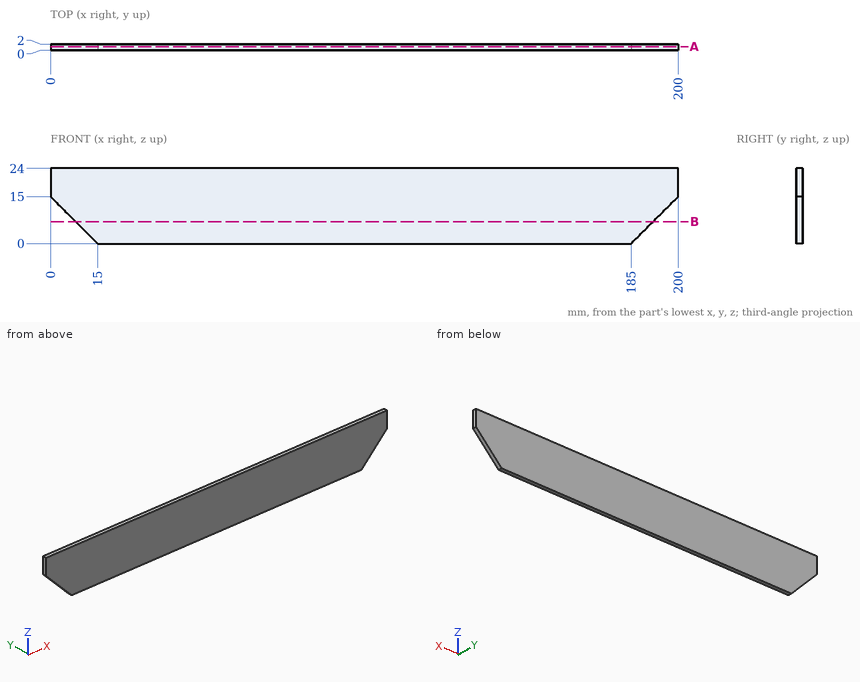
Print and shaded views of the part. All mm, measured from the part's lowest x, y and z. Give positions to 0.01 mm unless a question says otherwise; leave off trailing zeros. Loops run counter-clockwise (first coordinate to the right, second up) from the corner with the lowest first, then second, coordinate; pieces in that order, holes last.
1) Saw through at A-A (y = 1.15). Write the cut outline in (x, z), plus the area to 4 significant figures.
2) Saw through at B-B (z = 7). Write the cut outline in (x, y).
3) Wall check: line 1 (X direction, y = 1.2, z = 14); line 2 (Z direction, x = 14.5, y = 1.1); line 3 (X direction, y = 1.35, z = 10.5). Give the ranges that are in metal, low to high.
Answer block:
1. outline: (0, 15) - (15, 0) - (185, 0) - (200, 15) - (200, 24) - (0, 24) - close
1. area: 4,575 mm2
2. outline: (8, 0) - (192, 0) - (192, 2) - (8, 2) - close
3. line 1: x = 1 to 199
3. line 2: z = 0.5 to 24
3. line 3: x = 4.5 to 195.5
